```python
from build123d import *

# Parameters (mm, degrees)
F1_ANGLE = 90
F2_R     = 6.35
F3_DEPTH = 12.7
F3_TAPER = 5
F4_R     = 6.35
F5_DEPTH = 12.7
F5_TAPER = 5


with BuildPart() as f1:
    # F0 (on Front) → F1 (revolve)
    with BuildSketch(Plane.XZ):
        with BuildLine():
            Line((-108.4379373307, 138.5278597593), (-130.7680468253, 138.5278597593))
            ThreePointArc((-130.7680468253, 138.5278597593), (-155.8300717286, 109.5775467195), (-174.5961339778, 76.2))
            Line((-174.5961339778, 76.2), (-160.6437051366, 76.2))
            ThreePointArc((-160.6437051366, 76.2), (-163.4822477804, 69.9027514527), (-166.0740497489, 63.5))
            Line((-166.0740497489, 63.5), (-152.4, 63.5))
            ThreePointArc((-152.4, 63.5), (-149.5666310557, 69.9130379445), (-146.4635449523, 76.2))
            ThreePointArc((-146.4635449523, 76.2), (-111.6816124178, 121.5945206322), (-63.5, 152.4))
            Line((-63.5, 152.4), (-86.7975307453, 152.4))
            Line((-86.7975307453, 152.4), (-108.4379373307, 138.5278597593))
        make_face()
    revolve(axis=Axis((-5.3559339778, 0, 114.3), (0, 0, -1)), revolution_arc=F1_ANGLE)

    # F2 (on face) → F3 (join)
    with BuildSketch(Plane.XZ):
        with Locations((-146.7211129462, 100.4278597593)):
            Circle(F2_R)
    extrude(amount=F3_DEPTH, taper=F3_TAPER)

    # F4 (on face) → F5 (cut)
    with BuildSketch(Plane.YZ.offset(-5.3559339778)):
        with Locations((141.3651789683, 100.4278597593)):
            Circle(F4_R)
    extrude(amount=-F5_DEPTH, taper=F5_TAPER, mode=Mode.SUBTRACT)


solid = f1.part
```
Verification items for the finished model (mm, model axes). A direction names the side the tool comes from. Round coordinates to 2 decimals unless told otherwise and drop trailing zeros. Use CSV: the item, a comma, the result in double quotes.
(1) Gauge pin test, flat ends, axial feed: pin 1 Ø1 at (x, y) = (-124.5, 41) entering from +Z; pin 2 Ø5 at (y, z) = (142.5, 102.5) entering from +X; pin 3 Ø8 at (y, z) = (12.5, 142) entering from +X. Record the tip position at first contact, or that the pin passes through.
Entries:
pin 1,"z = 138.44"
pin 2,"x = -18.06"
pin 3,"x = -75.95"
(2) Access from +Z, -Z, +X, -X, +Y, -Y to the whole of each face (thin tool, end or side, straight path). Record for faces 5 (the face through (-82, 72, 138.528)), 6 (the face through (-5.356, 126, 108)).
Entries:
face 5,"+Z, -X, +Y"
face 6,"+Z, -Z, +X, +Y, -Y"
(3) Thickness scan on probe 1 along Z at (x, y) = (-154, 56.5); probe 2 along Z at (x, y) = (-57, 149); probe 3 along Z at (x, y) = (-55.5, 59). Record the ranges inside material, lowest first. Write a range as from..to.
Entries:
probe 1,"63.5..67.77, 76.2..96.29"
probe 2,"63.5..70.9, 76.2..98.51"
probe 3,"142.84..152.4"
(4) Mould release check, pull along Y, two halves, no side actions. Record for faces 1 (the face through (-108.4, 116.4, 76.2)), 2 (the face through (-66.26, 59.58, 149.99)), 3 (the face through (-11.79, 146.71, 98.21)), 4 (the face through (-18.056, 141, 101)): released by +Y, released by -Y, zero draft, split by the parting line, or undercut.
Entries:
face 1,"zero draft"
face 2,"released by +Y"
face 3,"undercut"
face 4,"undercut"
